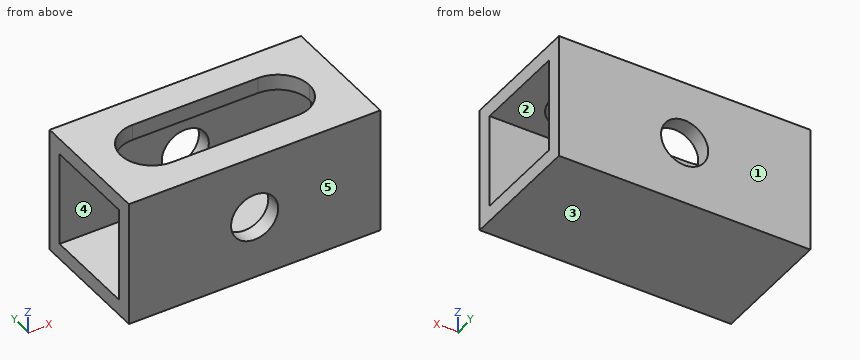
```python
from build123d import *

# Parameters (mm, degrees)
F0_W     = 50.8
F0_H     = 25.4
F1_DEPTH = 25.4
F2_W     = 19.05
F2_H     = 19.05
F3_DEPTH = 50.801
F4_R     = 4.7625
F5_DEPTH = 25.401
F7_DEPTH = 3.175


with BuildPart() as f1:
    # F0 (on Top) → F1 (new body)
    with BuildSketch(Plane.XY):
        with Locations((25.4, 12.7)):
            Rectangle(F0_W, F0_H)
    extrude(amount=F1_DEPTH)

    # F2 (on face) → F3 (cut, through all)
    with BuildSketch(Plane.YZ.offset(50.8)):
        with Locations((12.7, 12.7)):
            Rectangle(F2_W, F2_H)
    extrude(amount=-F3_DEPTH, mode=Mode.SUBTRACT)

    # F4 (on face) → F5 (cut, through all)
    with BuildSketch(Plane.XZ):
        with Locations((25.4, 12.7)):
            Circle(F4_R)
    extrude(amount=-F5_DEPTH, mode=Mode.SUBTRACT)

    # F6 (on face) → F7 (cut, through all)
    with BuildSketch(Plane.XY.offset(25.4)):
        with BuildLine():
            ThreePointArc((12.7, 19.05), (6.35, 12.7), (12.7, 6.35))
            Line((12.7, 6.35), (12.7, 19.05))
        make_face()
        with BuildLine():
            Line((12.7, 19.05), (12.7, 6.35))
            ThreePointArc((12.7, 6.35), (17.190128, 8.209872), (19.05, 12.7))
            ThreePointArc((19.05, 12.7), (17.190128, 17.190128), (12.7, 19.05))
        make_face()
        with BuildLine():
            Line((12.7, 6.35), (38.1, 6.35))
            ThreePointArc((38.1, 6.35), (31.75, 12.7), (38.1, 19.05))
            Line((38.1, 19.05), (12.7, 19.05))
            ThreePointArc((12.7, 19.05), (17.190128, 17.190128), (19.05, 12.7))
            ThreePointArc((19.05, 12.7), (17.190128, 8.209872), (12.7, 6.35))
        make_face()
        with BuildLine():
            ThreePointArc((38.1, 19.05), (31.75, 12.7), (38.1, 6.35))
            Line((38.1, 6.35), (38.1, 19.05))
        make_face()
        with BuildLine():
            Line((38.1, 19.05), (38.1, 6.35))
            ThreePointArc((38.1, 6.35), (42.590128, 8.209872), (44.45, 12.7))
            ThreePointArc((44.45, 12.7), (42.590128, 17.190128), (38.1, 19.05))
        make_face()
    extrude(amount=-F7_DEPTH, mode=Mode.SUBTRACT)


solid = f1.part
```
The listing builds one solid part. Answer for the finished solid, in the listing's coordinates (mm). Face numbers are marked on the shaded views. A direction names the side the tool comes from. Coordinates: 2 decimals unless noted, no trailing zeros. Write each loop counter-clockwise with the first axis right and the second up, starting at its lowest first coordinate (ties: lowest second). Pieces come first, ordered by that corner, then holes.
Q1. Section B-B, the plane z = 12.7 is taken. Write down the section's boundary in (x, y) (1 decimal).
Returned:
outline: (0, 0) - (20.6, 0) - (20.6, 3.2) - (0, 3.2) - close; (0, 22.2) - (20.6, 22.2) - (20.6, 25.4) - (0, 25.4) - close; (30.2, 0) - (50.8, 0) - (50.8, 3.2) - (30.2, 3.2) - close; (30.2, 22.2) - (50.8, 22.2) - (50.8, 25.4) - (30.2, 25.4) - close
Q2. Section D-D, the plane z = 22.75 is taken. Write down the section's boundary in (x, y).
Returned:
outline: (0, 0) - (50.8, 0) - (50.8, 25.4) - (0, 25.4) - close; hole (12.7, 6.35) - (38.1, 6.35) arc R6.35 ccw to (38.1, 19.05) - (12.7, 19.05) arc R6.35 ccw to start
Q3. Section C-C, the plane y = 20.75 is taken. Write down the section's boundary in (x, z) (3 decimals).
Returned:
outline: (0, 0) - (50.8, 0) - (50.8, 3.175) - (0, 3.175) - close; (0, 22.225) - (50.8, 22.225) - (50.8, 25.4) - (0, 25.4) - close
Q4. Find the intervals of material crossed by line 1 along Z through (x, y) = (43, 5.5) (3 decimals); line 2 along Y through (x, z) = (36, 22.75), in increasing order.
Returned:
line 1: z = 0 to 3.175, 22.225 to 25.4
line 2: y = 0 to 6.35, 19.05 to 25.4
Q5. Which of the six approach directions +Z, -Z, +X, -X, +Y, -Y give full straight-line access (tool end or side, diameter ignored) to the marked faces 4 and 5?
Returned:
face 4: +X, -X
face 5: +Z, -Z, +X, -X, -Y
Q6. Section A-A, the plane x = 4 is taken. Write down the section's boundary in (y, z) (3 decimals).
Returned:
outline: (0, 0) - (25.4, 0) - (25.4, 25.4) - (0, 25.4) - close; hole (3.175, 3.175) - (22.225, 3.175) - (22.225, 22.225) - (3.175, 22.225) - close
Q7. Given P1, Ø1, axis at x = 39, y = 16.5, coming from the +Z side (3 decimals), flat-ended and moving along its own axis, determine where the tip first touches the part or whether it passes through.
Returned:
P1: stops at z = 3.175
Q8. The mould has two halves that part along Z. Classify the marked faces 1, 2 and 3: released by +Z, released by -Z, zero draft, split by the parting line, or undercut.
Returned:
face 1: zero draft
face 2: undercut
face 3: released by -Z
